Autodesk Fusion 360 part; units mm, degrees
sketch "Sketch1" plane through (0, 0, 0) normal (0, 0, 1) x (1, 0, 0)
  arc A0 (40, 20.6155) -> (-40, 20.6155) centre (0, 0) ccw
  arc A1 (39.9116, 17.2383) -> (-40.1731, 16.7877) centre (-0.0351, 0.0189) ccw
  line L0 (-40, 20.6155) -> (-38.35, 20.6155)
  line L1 (40, 20.6155) -> (38.2797, 20.6155)
  line L2 (-40.1731, 16.7877) -> (-38.1731, 16.7877)
  line L3 (39.9116, 17.2383) -> (37.9116, 17.2383)
  line L4 (-36.35, 20.6155) -> (-38.1731, 16.7877)
  line L5 (36.2797, 20.6155) -> (37.9116, 17.2383)
  arc A2 (37.5794, 17.9258) -> (37.9116, 17.2383) centre (37.9116, 17.6623) ccw
  line L6 (35.69, 21.8359) -> (39.3471, 21.8359)
  line L7 (35.69, 21.8359) -> (36.2797, 20.6155)
  line L8 (-0.0351, 0.0189) -> (-0.0351, 49.45) construction
  line L9 (-35.7603, 21.8359) -> (-36.35, 20.6155)
  line L10 (-35.7603, 21.8359) -> (-39.4174, 21.8359)
  dimension "d2" = 80
  dimension "d4" = 2
  dimension "d5" = 2
  dimension "d6" = 2
  dimension "d7" = 2
extrude "Extrude1" add sketch "Sketch1" along normal blind 58 contours A0 A1 L1 L6 | A0 A1 L6 L10 | A1 L3 L5 L6 L7 | A0 A1 L0 L10 | A1 L2 L4 L9 L10
sketch "Sketch2" plane through (0, 0, 0) normal (0, 1, 0) x (1, 0, 0)
  line L0 (0, 0) -> (0, -5)
  line L1 (0, -5) -> (38, -5)
  line L2 (38, -5) -> (-38, -5)
  line L3 (-38, -5) -> (-38, -25)
  line L4 (-38, -25) -> (38, -25)
  line L5 (38, -25) -> (38, -5)
  line L6 (-8.3, -51) -> (11.7, -51)
  line L7 (11.7, -51) -> (11.7, -31)
  line L8 (11.7, -31) -> (-8.3, -31)
  line L9 (-8.3, -31) -> (-8.3, -51)
  line L10 (-8.3, -51) -> (11.7, -31) construction
  line L11 (11.7, -51) -> (-8.3, -31) construction
  line L12 (0, -57.95) -> (0, -50.95)
  point P0 (1.7, -41)
  dimension "d10" = 5
  dimension "d11" = 38
  dimension "d12" = 76
  dimension "d13" = 20
  dimension "d14" = 20
  dimension "d15" = 20
  dimension "d16" = 7
extrude "Extrude2" cut sketch "Sketch2" along normal blind 80
equation "d11 = ( 76 / 2 ) * 1 mm"
Design review of the part built by this model. Coordinates are the model's own, in mm. A direction names the side the tool comes from. Coordinates: 2 decimals unless noted, no trailing zeros. Order: outer loops, then holes, each group sorted by start corner. A loop starts at its lowest first (then second) coordinate and runs counter-clockwise, first axis right, second up. Notation, with made-up numbers: M 71,-18 L 110,-18 A16 cw 110,5 Z; hole C 57,51 d2. An arc over 180 degrees is marked long. Answer as a JSON object with one key per item and string values. Group by question number.
1) Add section C-C, the plane y = 25.5. Write out the cut boundary in (x, z).
2) Add section D-D, the plane x = 34.5. Write out the cut boundary in (y, z).
3) Add section B-B, the plane x = -6.5. Write out the cut boundary in (y, z), then the cut area to 3 significant figures.
4) Mouldability with a two-part tool opening along Z and no side actions: class faces 1 (the flat face through (2, 44, 31)), 2 (the flat face through (-37.25, 18.73, 35.04)), 3 (the flat face through (-0.3, 44.5, 0)), 4 (the flat face through (-0.3, 44.5, 58)) as pulls with the +Z half, pulls with the -Z half, needs draft (parallel to the pull), parting line crosses it, or undercut.
5) Wall thickness on L1, parallel to Y at x = 0, z = 27; L2, parallel to X at y = 31.5, z = 50; L3, parallel to X at y = 19.25, z = 37.5: over which ranges is each line inside the solid? List them lowest first.
6) Add section A-A, the plane z = 14. Write out the cut boundary in (x, y).
7) Tool access review of faces 5 (the flat face through (39, 17.238, 29)), 6 (the flat face through (11.7, 43, 41)), 7 (the cylindrical face through (-0.69, 44.995, 28.594)): name each direction out of +Z, -Z, +X, -X, +Y, -Y from which nothing blocks a thin tool from reaching the whole face with its end or side.
8) For pin 1 (10 mm diameter, centred on y = 39, z = 26.5, fed in from +X); pin 2 (0.6 mm diameter, centred on x = 37, z = 3.5, fed in from +Y); pin 3 (1.5 mm diameter, centred on y = 33, z = 29, fed in from -X), all flat-tipped, find the tip position at first contact; note any pin that passes through.
Computed values:
{
 "1": {"outline": "M -37.08,0 L -35.29,0 L -35.29,5 L -37.08,5 Z; M -37.08,25 L -35.29,25 L -35.29,58 L -37.08,58 Z; M 35.22,0 L 37.08,0 L 37.08,5 L 35.22,5 Z; M 35.22,25 L 37.08,25 L 37.08,58 L 35.22,58 Z"},
 "2": {"outline": "M 26.47,0 L 28.89,0 L 28.89,5 L 26.47,5 Z; M 26.47,25 L 28.89,25 L 28.89,58 L 26.47,58 Z"},
 "3": {"outline": "M 43.04,0 L 44.53,0 L 44.53,5 L 43.04,5 Z; M 43.04,25 L 44.53,25 L 44.53,31 L 43.04,31 Z; M 43.04,51 L 44.53,51 L 44.53,58 L 43.04,58 Z", "area": "26.9 mm^2"},
 "4": {"face 1": "undercut", "face 2": "needs draft", "face 3": "pulls with the -Z half", "face 4": "pulls with the +Z half"},
 "5": {"L1": "y = 43.52 to 45", "L2": "x = -32.14 to -30.05, 29.98 to 32.14", "L3": "x = -39.05 to -37, 36.94 to 38.98"},
 "6": {"outline": "M -40.17,16.79 L -38.17,16.79 L -38,17.15 L -38,24.1 A45 ccw -40,20.62 L -38.35,20.62 A43.5 ccw Z; M 38,17.24 L 39.91,17.24 A43.5 ccw 38.28,20.62 L 40,20.62 A45 ccw 38,24.1 Z"},
 "7": {"face 5": "+Z, -Z, +X, -Y", "face 6": "+Y, -Y", "face 7": "+Z, -Z, +Y"},
 "8": {"pin 1": "stops at x = 29.48", "pin 2": "stops at y = 26.04", "pin 3": "stops at x = -31.38"}
}
